Could you check a few things on this model? Use its own coordinates, in mm. A direction names the side the tool comes from. Coordinates: 2 decimals unless noted, no trailing zeros. Write each loop counter-clockwise with the first axis right and the second up, starting at its lowest first coordinate (ties: lowest second). Pieces come first, ordered by that corner, then holes.
Item 1: I want a section at B-B on y = -19. Please give me the cut outline in (x, z).
Item 2: Which directions (+Z, -Z, +X, -X, +Y, -Y) give clear straight access to the entire face, cutting with the end or side of a thin tool? Please do faces 1 (the flat face through (2, 8.953, 21)), 2 (the cylindrical face through (10.338, 1.142, 1.479)).
Item 3: Thinking about a two-plate mould opening in X: for faces 3 (the cylindrical face through (0.28, -27.81, 1.48)), 4 (the cylindrical face through (2.887, -38.042, 1.479)), 5 (the flat face through (7.2, -9, 3)), which applies, +X half, -X half, draft (parallel to the pull), parting line (faces both ways), or undercut?
Item 4: I want a section at C-C on z = 28. Please give me the cut outline in (x, y).
Item 5: For P1, Ø1, axis at x = 6, z = 31, coming from the -Y side; P2, Ø1.5, axis at x = -5, y = -32.5, coming from the +Z side; P3, Ø4, axis at x = 17.82, y = -11.06, coming from the -Z side, each with a flat end and sliding along its axis, tell me the tip position at first contact or that it passes through.
Item 6: I want a section at D-D on x = 4. Please give me the cut outline in (y, z), then the cut area to 3 significant figures.
Item 7: If I drill on probe 1 along Y at (x, z) = (-12.5, 4); probe 2 along Z at (x, y) = (14.5, -28); probe 3 along X at (y, z) = (-27, 2), over which ranges is the centre line in solid material (lowest first)?
Item 8: I want a section at A-A on x = 17.5. Please give me the cut outline in (y, z).
from build123d import *

# Parameters (mm, degrees)
SKETCH_1_R          = 10
EXTRUDE_2_DEPTH     = 40
CUT_EXTRUDE_START   = -37
CUT_EXTRUDE_1_DEPTH = 37
SKETCH_5_R          = 1.25
CUT_EXTRUDE_4_DEPTH = 3
SKETCH_6_R          = 1.25
CUT_EXTRUDE_5_DEPTH = 3
SKETCH_7_R          = 1.25
CUT_EXTRUDE_6_DEPTH = 3
SKETCH_8_R          = 1.25
CUT_EXTRUDE_7_DEPTH = 3


with BuildPart() as part:
    # 草图1 → 凸台-拉伸2 (new body)
    with BuildSketch(Plane.XY):
        with BuildLine():
            Line((-17.553025885, 11.952701951), (22.446974115, 11.952701951))
            Line((22.446974115, 11.952701951), (22.446974115, -18.047298049))
            ThreePointArc((22.446974115, -18.047298049), (2.446974115, -38.047298049), (-17.553025885, -18.047298049))
            Line((-17.553025885, -18.047298049), (-17.553025885, 11.952701951))
        make_face()
        with Locations((2.446974115, -18.047298049)):
            Circle(SKETCH_1_R, mode=Mode.SUBTRACT)
    extrude(amount=EXTRUDE_2_DEPTH)

    # 草图2 → 切除-拉伸1 (cut)
    with BuildSketch(Plane.XY.offset(40).offset(CUT_EXTRUDE_START)):
        with BuildLine():
            Line((-17.553025885, -18.047298049), (-17.553025885, 8.952701951))
            Line((-17.553025885, 8.952701951), (22.446974115, 8.952701951))
            Line((22.446974115, 8.952701951), (22.446974115, -18.047298049))
            ThreePointArc((22.446974115, -18.047298049), (2.446974115, -38.047298049), (-17.553025885, -18.047298049))
        make_face()
    extrude(amount=CUT_EXTRUDE_1_DEPTH, mode=Mode.SUBTRACT)

    # 草图5 → 切除-拉伸4 (cut)
    with BuildSketch(Plane(origin=(0, 0, 0), x_dir=(-1, 0, 0), z_dir=(0, 0, -1))):
        with Locations((-10.066616202, 2.362067463)):
            Circle(SKETCH_5_R)
    extrude(amount=-CUT_EXTRUDE_4_DEPTH, mode=Mode.SUBTRACT)

    # 草图6 → 切除-拉伸5 (cut)
    with BuildSketch(Plane(origin=(0, 0, 0), x_dir=(-1, 0, 0), z_dir=(0, 0, -1))):
        with Locations((5.433383798, 2.362067463)):
            Circle(SKETCH_6_R)
    extrude(amount=-CUT_EXTRUDE_5_DEPTH, mode=Mode.SUBTRACT)

    # 草图7 → 切除-拉伸6 (cut)
    with BuildSketch(Plane(origin=(0, 0, 0), x_dir=(-1, 0, 0), z_dir=(0, 0, -1))):
        with Locations((-17.816616202, -11.061326295)):
            Circle(SKETCH_7_R)
    extrude(amount=-CUT_EXTRUDE_6_DEPTH, mode=Mode.SUBTRACT)

    # 草图8 → 切除-拉伸7 (cut)
    with BuildSketch(Plane(origin=(0, 0, 0), x_dir=(-1, 0, 0), z_dir=(0, 0, -1))):
        with Locations((13.183383798, -11.061326295)):
            Circle(SKETCH_8_R)
    extrude(amount=-CUT_EXTRUDE_7_DEPTH, mode=Mode.SUBTRACT)


solid = part.part
Response values:
1. outline: (-17.53, 0) - (-7.51, 0) - (-7.51, 3) - (-17.53, 3) - close; (12.4, 0) - (22.42, 0) - (22.42, 3) - (12.4, 3) - close
2. face 1: +Z, +X, -X, -Y
2. face 2: +Z, -Z
3. face 3: undercut
3. face 4: parting line
3. face 5: draft
4. outline: (-17.55, 8.95) - (22.45, 8.95) - (22.45, 11.95) - (-17.55, 11.95) - close
5. P1: stops at y = 8.95
5. P2: stops at z = 3
5. P3: stops at z = 0
6. outline: (-37.99, 0) - (-27.93, 0) - (-27.93, 3) - (-37.99, 3) - close; (-8.17, 0) - (11.95, 0) - (11.95, 40) - (8.95, 40) - (8.95, 3) - (-8.17, 3) - close
6. area: 202 mm2
7. probe 1: y = 8.95 to 11.95
7. probe 2: z = 0 to 3
7. probe 3: x = -15.44 to -2.01, 6.9 to 20.33
8. outline: (-31.22, 0) - (-12.27, 0) - (-12.27, 3) - (-31.22, 3) - close; (-9.85, 0) - (11.95, 0) - (11.95, 40) - (8.95, 40) - (8.95, 3) - (-9.85, 3) - close
